Autodesk Inventor part; units mm, degrees
ref_plane "YZ Plane" through (0, 0, 0) normal (1, 0, 0) x (0, 1, 0)
ref_plane "XZ Plane" through (0, 0, 0) normal (0, 1, 0) x (-1, 0, 0)
ref_plane "XY Plane" through (0, 0, 0) normal (0, 0, 1) x (1, 0, 0)
ref_plane "Work Plane1" through (0, 0, 0) normal (0, 0, 1) x (1, 0, 0)
sketch "Sketch1" plane through (0, 0, 0) normal (0, 0, 1) x (1, 0, 0)
  line L0 (-9.25, 7.625) -> (-9.25, -7.625)
  line L1 (-9.25, -7.625) -> (-29.75, -7.625)
  line L2 (-29.75, -7.625) -> (-29.75, -29.875)
  line L3 (-29.75, -29.875) -> (0, -29.875)
  line L4 (0, -29.875) -> (0, 29.875)
  line L5 (0, 29.875) -> (-29.75, 29.875)
  line L6 (-29.75, 29.875) -> (-29.75, 7.625)
  line L7 (-29.75, 7.625) -> (-9.25, 7.625)
  circle A0 centre (-15, 14.875) radius 3.5
  circle A1 centre (-15, -14.875) radius 3.5
  circle A2 centre (-7, 20) radius 1.35
  circle A3 centre (-6, 0) radius 1.35
  circle A4 centre (-7, -20) radius 1.35
  circle A5 centre (-22.75, -20) radius 1.35
  circle A6 centre (-22.75, 20) radius 1.35
  line L8 (-29.75, -29.875) -> (0, -29.875)
  line L9 (0, 29.875) -> (-29.75, 29.875)
  point P0 (0, 0)
extrude "Extrusion1" add sketch "Sketch1" along normal blind 25.2 contours L7 L6 L5 L4 L3 L2 L1 L0 | A0 | A1 | A3
sketch "Sketch3" plane through (0, -29.875, 0) normal (1, 0, 0) x (0, 0, -1)
  circle A0 centre (-12.6232, 29.875) radius 1.621
  point P0 (0, 29.875)
hole "Hole2" at (0, 0, 12.6232) direction (-1, 0, 0) diameter 3.242 depth 6
properties part number "holder1"
Can you work these out from the model? Positions are in its coordinate system, mm. A direction names the side the tool comes from. Coordinates: 2 decimals unless noted, no trailing zeros. Loops run counter-clockwise (first coordinate to the right, second up) from the corner with the lowest first, then second, coordinate; pieces in that order, holes last. Notation, with made-up numbers: (10, 83) - (42, 83) arc R27 ccw to (42, 112) - close; hole circle Ø4 at (10, -24). An arc over 180 degrees is marked (long way). Answer as CSV lines item,"result". Start each with the question number.
1) For pin 1 (4 mm diameter, centred on y = 0, z = 12.62, fed in from -X), with a flat end and sliding along its axis, tell me the tip position at first contact or that it passes through.
2) Suppose I cut it at B-B (x = -22.75). Please give me the cut outline in (y, z) (3 decimals).
3) I need wall thicknesses on line 1 (Y direction, x = -7, z = 9.25) (3 decimals); line 2 (Y direction, x = -15, z = 11.5) (3 decimals); line 3 (Y direction, x = -6.25, z = 12.5) (1 decimal). Which ranges of each line are inside material? Lowest first, please. Write a range as from..to.
4) Which directions (+Z, -Z, +X, -X, +Y, -Y) give clear straight access to the entire face, cutting with the end or side of a thin tool? Please do faces 5 (the flat face through (-19, -7.625, 12)), 6 (the flat face through (-6, 0, 13)), 7 (the flat face through (-29.75, 19, 12)).
5) Suppose I cut it at A-A (y = -20). Please give me the cut outline in (x, z).
6) Suppose I cut it at D-D (x = -26). Please give me the cut outline in (y, z) (3 decimals), plus the area to 3 significant figures.
7) Thinking about a two-plate mould opening in X: for faces 1 (the cylindrical face through (-5.753, -19.483, 12.424)), 2 (the cylindrical face through (-5.753, 20.517, 12.424)), 3 (the flat face through (-29.75, -19, 12)), 4 (the flat face through (-20, 7.625, 12)), which applies, pulls with the +X half, pulls with the -X half, needs draft (parallel to the pull), parting line crosses it, or undercut?
8) Suppose I cut it at C-C (z = 3.5). Please give me the cut outline in (x, y) (3 decimals).
Check result:
1,pin 1,"stops at x = -9.25"
2,outline,"(-29.875, 0) - (-21.35, 0) - (-21.35, 25.2) - (-29.875, 25.2) - close; (-18.65, 0) - (-7.625, 0) - (-7.625, 25.2) - (-18.65, 25.2) - close; (7.625, 0) - (18.65, 0) - (18.65, 25.2) - (7.625, 25.2) - close; (21.35, 0) - (29.875, 0) - (29.875, 25.2) - (21.35, 25.2) - close"
3,line 1,"y = -29.875..-21.35, -18.65..18.65, 21.35..29.875"
3,line 2,"y = -29.875..-7.625, 7.625..29.875"
3,line 3,"y = -29.9..-21.1, -18.9..18.9, 21.1..29.9"
4,face 5,"+Z, -Z, -X"
4,face 6,"+X"
4,face 7,"+Z, -Z, -X, +Y, -Y"
5,outline,"(-29.75, 0) - (-24.1, 0) - (-24.1, 25.2) - (-29.75, 25.2) - close; (-21.4, 0) - (-8.35, 0) - (-8.35, 25.2) - (-21.4, 25.2) - close; (-5.65, 0) - (0, 0) - (0, 25.2) - (-5.65, 25.2) - close"
6,outline,"(-29.875, 0) - (-7.625, 0) - (-7.625, 25.2) - (-29.875, 25.2) - close; (7.625, 0) - (29.875, 0) - (29.875, 25.2) - (7.625, 25.2) - close"
6,area,"1,120 mm²"
7,face 1,"undercut"
7,face 2,"undercut"
7,face 3,"pulls with the -X half"
7,face 4,"needs draft"
8,outline,"(-29.75, -29.875) - (0, -29.875) - (0, 29.875) - (-29.75, 29.875) - (-29.75, 7.625) - (-9.25, 7.625) - (-9.25, -7.625) - (-29.75, -7.625) - close; hole circle Ø2.7 at (-22.75, -20); hole circle Ø2.7 at (-22.75, 20); hole circle Ø2.7 at (-7, -20); hole circle Ø2.7 at (-7, 20)"
